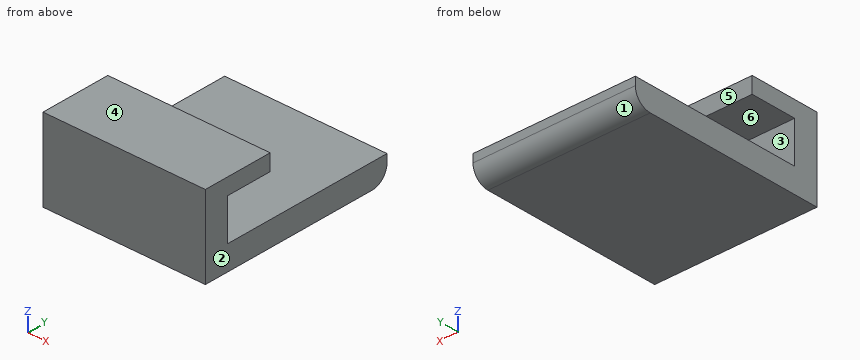
```python
from build123d import *

# Parameters (mm, degrees)
F1_DEPTH = 20


with BuildPart() as f1:
    # F0 (on Right) → F1 (new body)
    with BuildSketch(Plane.YZ):
        with BuildLine():
            Line((-23.957143, -5.842857), (-1.575925, -5.842857))
            ThreePointArc((-1.575925, -5.842857), (-0.161711, -5.257071), (0.424075, -3.842857))
            Line((0.424075, -3.842857), (0.424075, -2.842857))
            Line((0.424075, -2.842857), (-20.957143, -2.842857))
            Line((-20.957143, -2.842857), (-20.957143, 2.257143))
            Line((-20.957143, 2.257143), (-15.257143, 2.257143))
            Line((-15.257143, 2.257143), (-15.257143, 4.257143))
            Line((-15.257143, 4.257143), (-23.957143, 4.257143))
            Line((-23.957143, 4.257143), (-23.957143, -5.842857))
        make_face()
    extrude(amount=F1_DEPTH)


solid = f1.part
```
Input: part model. Units: mm. Frame: model coordinates. Face numbers are marked on the shaded views. A direction names the side the tool comes from. Round coordinates to 2 decimals unless told otherwise and drop trailing zeros. Loops run counter-clockwise (first coordinate to the right, second up) from the corner with the lowest first, then second, coordinate; pieces in that order, holes last. Notation, with made-up numbers: (-2, -8) -> (3, -8) arc R24 ccw to (3, 23) -> close; hole circle Ø3 at (43, 4.25). An arc over 180 degrees is marked (long way). Use one line per item in the form item = value. Start each with the question number.
Item 1: Contact query for flat-ended pins moving along their axis: pin 1 Ø1 at (x, z) = (9, 3.5) entering from +Y; pin 2 Ø1.5 at (x, z) = (12.5, 0.5) entering from +Y; pin 3 Ø3 at (x, y) = (3.5, -11) entering from +Z. Output: stop coordinate, or through.
Item 2: Set-up query: the marked faces 4, 5 and 6. Return all of +Z, -Z, +X, -X, +Y, -Y with unobstructed straight access to the full face (end or side cutting, diameter ignored); none if empty.
Item 3: Section query A-A on y = -19.25. Return the cut outline in (x, z), then the cut area to 3 significant figures.
Item 4: Mould query, pull axis Z, two halves, no side actions, for the marked faces 1, 2 and 3. Classes: pulls with the +Z half, pulls with the -Z half, needs draft (parallel to the pull), parting line crosses it, or undercut.
Item 5: Section query B-B on x = 7. Return the cut outline in (y, z), then the cut area to 3 significant figures.
Item 6: Material intervals for L1, parallel to Z at x = 8.5, y = -18.75; L2, parallel to Z at x = 11, y = -4.25; L3, parallel to Y at x = 8.5, z = 2, sorted ascending. Write a range as from..to.
Item 7: Section query C-C on z = 3.5. Return the cut outline in (x, y), then the cut area to 3 significant figures.
Item 8: Section query D-D on y = -3.5. Return the cut outline in (x, z).
Ans:
q1.pin_1 = -15.26
q1.pin_2 = -20.96
q1.pin_3 = -2.84
q2.face_4 = +Z, +X, -X, +Y, -Y
q2.face_5 = +Z, +X, -X, +Y
q2.face_6 = +X, -X, +Y
q3.outline = (0, -5.84) -> (20, -5.84) -> (20, -2.84) -> (0, -2.84) -> close; (0, 2.26) -> (20, 2.26) -> (20, 4.26) -> (0, 4.26) -> close
q3.area = 100 mm^2
q4.face_1 = pulls with the -Z half
q4.face_2 = needs draft
q4.face_3 = undercut
q5.outline = (-23.96, -5.84) -> (-1.58, -5.84) arc R2 ccw to (0.42, -3.84) -> (0.42, -2.84) -> (-20.96, -2.84) -> (-20.96, 2.26) -> (-15.26, 2.26) -> (-15.26, 4.26) -> (-23.96, 4.26) -> close
q5.area = 105 mm^2
q6.L1 = -5.84..-2.84, 2.26..4.26
q6.L2 = -5.84..-2.84
q6.L3 = -23.96..-20.96
q7.outline = (0, -23.96) -> (20, -23.96) -> (20, -15.26) -> (0, -15.26) -> close
q7.area = 174 mm^2
q8.outline = (0, -5.84) -> (20, -5.84) -> (20, -2.84) -> (0, -2.84) -> close
